Geometry check sheet. Reference: drawing and pictorial views, mm from the part's lowest x, y, z. Coordinates: 2 decimals unless noted, no trailing zeros. Write each loop counter-clockwise with the first axis right and the second up, starting at its lowest first coordinate (ties: lowest second). Pieces come first, ordered by that corner, then holes. Notation, with made-up numbers: (59, 32.5) -> (118, 32.5) arc R30 cw to (118, 63.5) -> close; hole circle Ø1 at (81, -18). An arc over 180 degrees is marked (long way). Use a Markdown table: item, result.
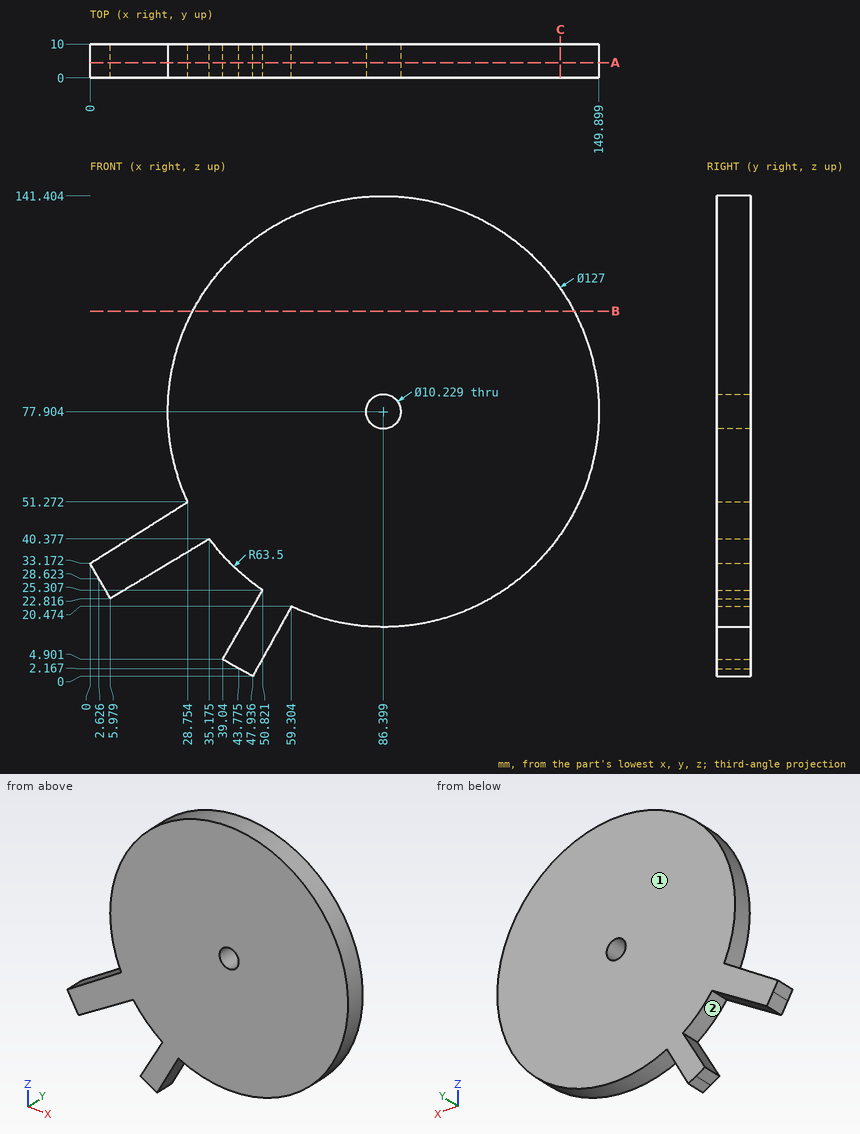
Item 1: Section check A-A on y = 4.5. Record the boundary of the cut face in (x, z) (1 decimal).
Answer block:
| item | result |
|---|---|
| outline | (0, 33.2) -> (6, 22.8) -> (35.2, 40.4) arc R63.5 ccw to (50.8, 25.3) -> (39, 4.9) -> (43.8, 2.2) -> (47.9, 0) -> (59.3, 20.5) arc R63.5 ccw (long way) to (28.8, 51.3) -> close; hole circle Ø10.2 at (86.4, 77.9) |
Item 2: Depth check by flat-ended pin: P1, Ø5, axis at y = 4, z = 65, coming from the -X side; P2, Ø5, axis at y = 3, z = 46.5, coming from the -X side; P3, Ø5, axis at x = 78, y = 3.5, coming from the -Z side. Enter the tip coordinate at first touch or a pass-through.
Answer block:
| item | result |
|---|---|
| P1 | stops at x = 23.76 |
| P2 | stops at x = 17.2 |
| P3 | stops at z = 14.68 |
Item 3: Thickness scan on L1, parallel to Z at x = 28, y = 4.75 (1 decimal); L2, parallel to X at y = 0.5, z = 80 (1 decimal); L3, parallel to X at y = 3.5, z = 81 (1 decimal). Record the ranges inside material, lowest first. Write a range as [from, to].
Answer block:
| item | result |
|---|---|
| L1 | z = [36.1, 50.8], [53, 102.8] |
| L2 | x = [22.9, 81.7], [91.1, 149.9] |
| L3 | x = [23, 82.3], [90.5, 149.8] |
Item 4: Section check B-B on z = 107.5. Record the boundary of the cut face in (x, y), then the cut area to 3 significant figures.
Answer block:
| item | result |
|---|---|
| outline | (30.22, 0) -> (142.58, 0) -> (142.58, 10) -> (30.22, 10) -> close |
| area | 1,120 mm^2 |
Item 5: Mould release check, pull along X, two halves, no side actions. Record for the marked faces 1 and 2: +X half, -X half, draft (parallel to the pull), parting line (faces both ways), or undercut.
Answer block:
| item | result |
|---|---|
| face 1 | draft |
| face 2 | undercut |
Item 6: Section check C-C on x = 138.5. Record the boundary of the cut face in (y, z) (1 decimal).
Answer block:
| item | result |
|---|---|
| outline | (0, 41.6) -> (10, 41.6) -> (10, 114.2) -> (0, 114.2) -> close |
